from build123d import *

# Parameters (mm, degrees)
SKETCH_1_W                  = 320
SKETCH_1_H                  = 200
EXTRUDE_1_DEPTH             = 237
SKETCH_2_R                  = 11
CUT_EXTRUDE_1_DEPTH         = 446.610816745
PATTERN_LINEAR_1_COUNT      = 4
PATTERN_LINEAR_1_PITCH      = 80
PATTERN_LINEAR_1_COUNT_DIR2 = 2
PATTERN_LINEAR_1_PITCH_DIR2 = 110
SKETCH_6_W                  = 211
SKETCH_6_H                  = 93.5
CUT_EXTRUDE_3_DEPTH         = 446.610816745
SKETCH_7_R                  = 25
CUT_EXTRUDE_4_DEPTH         = 413.202923328


with BuildPart() as part:
    # 草图1 → 拉伸1 (new body)
    with BuildSketch(Plane.XY):
        with Locations((160, 100)):
            Rectangle(SKETCH_1_W, SKETCH_1_H)
    extrude(amount=EXTRUDE_1_DEPTH)

    # 草图2 → 切除-拉伸1 (cut, through all)
    with BuildSketch(Plane.XY.offset(237)):
        with Locations((40, 45)):
            Circle(SKETCH_2_R)
    cut_extrude_1 = extrude(amount=-CUT_EXTRUDE_1_DEPTH, mode=Mode.SUBTRACT)

    # 阵列(线性)1: Cut-Extrude 1 4 × 2
    with Locations(*[(i * PATTERN_LINEAR_1_PITCH, j * PATTERN_LINEAR_1_PITCH_DIR2, 0) for i in range(PATTERN_LINEAR_1_COUNT) for j in range(PATTERN_LINEAR_1_COUNT_DIR2) if (i, j) != (0, 0)]):
        add(cut_extrude_1, mode=Mode.SUBTRACT)

    # 草图6 → 切除-拉伸3 (cut, through all)
    with BuildSketch(Plane.ZY):
        with Locations((118.5, 153.25)):
            Rectangle(SKETCH_6_W, SKETCH_6_H)
        with Locations((118.5, 46.75)):
            Rectangle(SKETCH_6_W, SKETCH_6_H)
    extrude(amount=-CUT_EXTRUDE_3_DEPTH, mode=Mode.SUBTRACT)

    # 草图7 → 切除-拉伸4 (cut, through all)
    with BuildSketch(Plane(origin=(0, 106.5, 0), x_dir=(1, 0, 0), z_dir=(0, 1, 0))):
        with Locations(Location((160, -118.5, 0), (0, 0, 270))):
            Circle(SKETCH_7_R)
    extrude(amount=-CUT_EXTRUDE_4_DEPTH, mode=Mode.SUBTRACT)


solid = part.part
Could you check a few things on this model? Use its own coordinates, in mm. A direction names the side the tool comes from. Coordinates: 2 decimals unless noted, no trailing zeros. Order: outer loops, then holes, each group sorted by start corner. A loop starts at its lowest first (then second) coordinate and runs counter-clockwise, first axis right, second up.
Q1. Please list where these lines run through material, in increasing order: L1, parallel to Y at x = 200, z = 8; L2, parallel to Z at x = 66.5, y = 21; L3, parallel to Y at x = 184.5, z = 196.5.
Q2. Suppose I cut it at B-B on x = 245. Please give me the cut outline in (y, z).
Q3. Thinking about a two-plate mould opening in Y: for faces 1 (the flat face through (158, 153, 13)), 2 (the cylindrical face through (269, 45, 7)), 3 (the flat face through (158, 0, 6)), 4 (the cylindrical face through (38.568, 165.906, 6.591)), which applies, released by +Y, released by -Y, zero draft, split by the parting line, or undercut?
Q4. Suppose I cut it at C-C on x = 120. Please give me the cut outline in (y, z).
Q5. Suppose I cut it at A-A on y = 118.5. Please give me the cut outline in (x, z), and give its area (3 significant figures).
Q6. Will these pins go through, and if not, where does the flat tip stop? pin 1 (20 mm diameter, centred on x = 280, y = 155, fed in from -Z); pin 2 (5 mm diameter, centred on x = 103.5, z = 62, fed in from -Y); pin 3 (2 mm diameter, centred on x = 177, z = 81.5, fed in from +Y).
Q7. Suppose I cut it at D-D on y = 45. Give the number of separate pieces and of enclosed holes in the cut face, and give its area (3 significant figures).
Q8. Which directions (+Z, -Z, +X, -X, +Y, -Y) give clear straight access to the entire face, cutting with the end or side of a thin tool? Please do faces 5 (the cylindrical face through (191.89, 162.43, 230.59)), 6 (the flat face through (193, 106.5, 117)), 7 (the flat face through (193, 93.5, 117)).
Answer:
1. L1: y = 0 to 34, 56 to 144, 166 to 200
1. L2: z = 0 to 13, 224 to 237
1. L3: y = 93.5 to 106.5
2. outline: (0, 0) - (200, 0) - (200, 13) - (106.5, 13) - (106.5, 224) - (200, 224) - (200, 237) - (0, 237) - (0, 224) - (93.5, 224) - (93.5, 13) - (0, 13) - close
3. face 1: zero draft
3. face 2: undercut
3. face 3: released by -Y
3. face 4: undercut
4. outline: (0, 0) - (34, 0) - (34, 13) - (0, 13) - close; (0, 224) - (34, 224) - (34, 237) - (0, 237) - close; (56, 0) - (144, 0) - (144, 13) - (106.5, 13) - (106.5, 224) - (144, 224) - (144, 237) - (56, 237) - (56, 224) - (93.5, 224) - (93.5, 13) - (56, 13) - close; (166, 0) - (200, 0) - (200, 13) - (166, 13) - close; (166, 224) - (200, 224) - (200, 237) - (166, 237) - close
5. outline: (0, 0) - (320, 0) - (320, 13) - (0, 13) - close; (0, 224) - (320, 224) - (320, 237) - (0, 237) - close
5. area: 8,320 mm2
6. pin 1: passes through
6. pin 2: stops at y = 93.5
6. pin 3: stops at y = 106.5
7. separate pieces: 10
7. enclosed holes: 0
7. area: 6,030 mm2
8. face 5: +Z, -Z
8. face 6: +X, -X, +Y
8. face 7: +X, -X, -Y
